from build123d import *

# Parameters (mm, degrees)
SKETCH1_W           = 68
SKETCH1_H           = 54
BOSS_EXTRUDE1_DEPTH = 8
CUT_EXTRUDE1_DEPTH  = 51
SKETCH2_3_W         = 28.5
SKETCH2_3_H         = 2.140954579
SKETCH2_3_W_2       = 28
CUT_EXTRUDE2_DEPTH  = 65.311740763
FILLET1_R           = 3
FILLET2_R           = 3
SKETCH3_W           = 40
SKETCH3_H           = 2.334194627
CUT_EXTRUDE3_DEPTH  = 51
FILLET3_R           = 3
FILLET4_R           = 3
FILLET5_R           = 3
SKETCH1_3_W         = 8
SKETCH1_3_H         = 8
SKETCH1_3_R         = 1.55
BOSS_EXTRUDE2_DEPTH = 3
FILLET6_R           = 3
FILLET7_R           = 1
FILLET8_R           = 1
FILLET9_R           = 1


with BuildPart() as part:
    # Sketch1 → Boss-Extrude1 (new body)
    with BuildSketch(Plane(origin=(0, 0, 0), x_dir=(1, 0, 0), z_dir=(0, 1, 0))):
        Rectangle(SKETCH1_W, SKETCH1_H)
    extrude(amount=BOSS_EXTRUDE1_DEPTH)

    # Sketch2 → Cut-Extrude1 (cut)
    with BuildSketch(Plane(origin=(0, 0, -27), x_dir=(-1, 0, 0), z_dir=(0, 0, -1))):
        Polygon((-30.5, 2.334194627), (0, 2.334194627), (0, 5.859045421), (-28.5, 5.859045421), (-30.5, 5.859045421), align=None)
        Polygon((0, 5.859045421), (0, 2.334194627), (30, 2.334194627), (30, 5.859045421), (28, 5.859045421), align=None)
    extrude(amount=-CUT_EXTRUDE1_DEPTH, mode=Mode.SUBTRACT)

    # Sketch2<3> → Cut-Extrude2 (cut, through all)
    with BuildSketch(Plane(origin=(0, 0, -27), x_dir=(-1, 0, 0), z_dir=(0, 0, -1))):
        with Locations((-14.25, 6.929522711)):
            Rectangle(SKETCH2_3_W, SKETCH2_3_H)
        with Locations((14, 6.929522711)):
            Rectangle(SKETCH2_3_W_2, SKETCH2_3_H)
    extrude(amount=-CUT_EXTRUDE2_DEPTH, mode=Mode.SUBTRACT)

    # Fillet1
    # the kernel refuses this fillet: 3 mm, written as the material it adds along each edge
    with BuildSketch(Plane(origin=(30.5, 5.859045421, -27), x_dir=(0, -1, 0), z_dir=(0, 0, 1))) as fillet1_piece_1:
        with BuildLine():
            CenterArc((2.828427125, -3), FILLET1_R, 90, 70.528779366)
            Line((0, -2), (-0.056568542, -1.98))
            ThreePointArc((-0.056568542, -1.98), (-0.06, -1), (-0.06, 0))
            Line((-0.06, 0), (0, 0.06))
            Line((0, 0.06), (2.828427125, 0.06))
            Line((2.828427125, 0.06), (2.828427125, 0))
        make_face()
    extrude(amount=51)
    with BuildSketch(Plane(origin=(-30, 5.859045421, -27), x_dir=(1, 0, 0), z_dir=(0, 0, 1))) as fillet1_piece_2:
        with BuildLine():
            CenterArc((3, -2.828427125), FILLET1_R, 109.471220634, 70.528779366)
            Line((0, -2.828427125), (-0.06, -2.828427125))
            Line((-0.06, -2.828427125), (-0.06, 0))
            Line((-0.06, 0), (0, 0.06))
            ThreePointArc((0, 0.06), (1, 0.06), (1.98, 0.056568542))
            Line((1.98, 0.056568542), (2, 0))
        make_face()
    extrude(amount=51)

    # Fillet2
    fillet2_edges = [part.edges().sort_by_distance(p)[0] for p in [
        (34, 8, 0),
        (-34, 8, 0),
    ]]
    fillet(fillet2_edges, radius=FILLET2_R)

    # Sketch3 → Cut-Extrude3 (cut)
    with BuildSketch(Plane(origin=(0, 0, -27), x_dir=(-1, 0, 0), z_dir=(0, 0, -1))):
        with Locations((0, 1.167097314)):
            Rectangle(SKETCH3_W, SKETCH3_H)
    extrude(amount=-CUT_EXTRUDE3_DEPTH, mode=Mode.SUBTRACT)

    # Fillet3
    fillet3_edges = [part.edges().sort_by_distance(p)[0] for p in [
        (20, 1.167097313, 24),
        (-20, 1.167097313, 24),
    ]]
    fillet(fillet3_edges, radius=FILLET3_R)

    # Fillet4
    # the kernel refuses this fillet: 3 mm, written as the material it takes off along each edge
    with BuildSketch(Plane(origin=(-17, 2.334194627, 21), x_dir=(0.6464786745536378, 0, -0.762932056835582), z_dir=(-0.762932056835582, 0, -0.6464786745536378))) as fillet4_piece_1_section:
        with BuildLine():
            CenterArc((5.925184303, 3), FILLET4_R, 192.822717627, 77.177282373)
            Line((3, 2.334194627), (3, 0))
            Line((3, 0), (5.925184303, 0))
        make_face()
    fillet4_piece_1 = revolve(axis=Axis((-17, 2.334194627, 21), (0, -1, 0)), revolution_arc=229.72336785, mode=Mode.PRIVATE)
    fillet4_piece_1 = split(fillet4_piece_1, bisect_by=Plane(origin=(-17, 2.334194627, 24), z_dir=(0, 0, -1)), keep=Keep.TOP, mode=Mode.PRIVATE)
    add(fillet4_piece_1, mode=Mode.SUBTRACT)
    with BuildSketch(Plane(origin=(17, 2.334194627, 21), x_dir=(1, 0, 0), z_dir=(0, 0, -1))) as fillet4_piece_2_section:
        with BuildLine():
            CenterArc((5.925184303, 3), FILLET4_R, 192.822717627, 77.177282373)
            Line((3, 2.334194627), (3, 0))
            Line((3, 0), (5.925184303, 0))
        make_face()
    fillet4_piece_2 = revolve(axis=Axis((17, 2.334194627, 21), (0, -1, 0)), revolution_arc=229.72336785, mode=Mode.PRIVATE)
    fillet4_piece_2 = split(fillet4_piece_2, bisect_by=Plane(origin=(17, 2.334194627, 24), z_dir=(0, 0, -1)), keep=Keep.TOP, mode=Mode.PRIVATE)
    add(fillet4_piece_2, mode=Mode.SUBTRACT)
    with BuildSketch(Plane(origin=(-20, 2.334194627, -34.312960757), x_dir=(-1, 0, 0), z_dir=(0, 0, 1))) as fillet4_piece_3:
        with BuildLine():
            CenterArc((2.925184303, 3), FILLET4_R, 192.822717627, 77.177282373)
            Line((0, 2.334194627), (0, 0))
            Line((0, 0), (2.925184303, 0))
        make_face()
    extrude(amount=55.312960757, mode=Mode.SUBTRACT)
    with BuildSketch(Plane(origin=(20, 2.334194627, -34.312960757), x_dir=(1, 0, 0), z_dir=(0, 0, 1))) as fillet4_piece_4:
        with BuildLine():
            CenterArc((2.925184303, -3), FILLET4_R, 90, 77.177282373)
            Line((0, -2.334194627), (0, 0))
            Line((0, 0), (2.925184303, 0))
        make_face()
    extrude(amount=55.312960757, mode=Mode.SUBTRACT)

    # Fillet5
    # the kernel refuses this fillet: 3 mm, written as the material it adds along each edge
    with BuildSketch(Plane(origin=(28.5, 5.859045421, 24), x_dir=(-1, 0, 0), z_dir=(0, 0, 1))) as fillet5_piece_1:
        with BuildLine():
            CenterArc((2.874376622, -3), FILLET5_R, 90, 73.360529794)
            Line((0, -2.140954579), (-0.057487532, -2.123773671))
            ThreePointArc((-0.057487532, -2.123773671), (-0.06, -1.07047729), (-0.06, 0))
            Line((-0.06, 0), (0, 0.06))
            Line((0, 0.06), (2.874376622, 0.06))
            Line((2.874376622, 0.06), (2.874376622, 0))
        make_face()
    extrude(amount=3)
    with BuildSketch(Plane(origin=(-28, 5.859045421, 24), x_dir=(1, 0, 0), z_dir=(0, 0, 1))) as fillet5_piece_2:
        with BuildLine():
            CenterArc((2.874376622, 3), FILLET5_R, 196.639470206, 73.360529794)
            Line((0, 2.140954579), (-0.057487532, 2.123773671))
            ThreePointArc((-0.057487532, 2.123773671), (-0.06, 1.07047729), (-0.06, 0))
            Line((-0.06, 0), (0, -0.06))
            Line((0, -0.06), (2.874376622, -0.06))
            Line((2.874376622, -0.06), (2.874376622, 0))
        make_face()
    extrude(amount=3)

    # Sketch1<3> → Boss-Extrude2 (add)
    # profile 1 of 2: a face of its own
    with BuildSketch(Plane(origin=(0, 0, 0), x_dir=(1, 0, 0), z_dir=(0, 1, 0))):
        with Locations((-38, 0)):
            Rectangle(SKETCH1_3_W, SKETCH1_3_H)
        with Locations(Location((-38, 0, 0), (0, 0, 270))):
            Circle(SKETCH1_3_R, mode=Mode.SUBTRACT)
    # profile 2 of 2: a face of its own
    with BuildSketch(Plane(origin=(0, 0, 0), x_dir=(1, 0, 0), z_dir=(0, 1, 0))):
        with Locations((38, 0)):
            Rectangle(SKETCH1_3_W, SKETCH1_3_H)
        with Locations(Location((38, 0, 0), (0, 0, 270))):
            Circle(SKETCH1_3_R, mode=Mode.SUBTRACT)
    extrude(amount=BOSS_EXTRUDE2_DEPTH)

    # Fillet6
    fillet6_edges = [part.edges().sort_by_distance(p)[0] for p in [
        (-34, 1.5, -4),
        (-34, 1.5, 4),
        (34, 1.5, -4),
        (34, 1.5, 4),
    ]]
    fillet(fillet6_edges, radius=FILLET6_R)

    # Fillet7
    fillet7_edges = [part.edges().sort_by_distance(p)[0] for p in [
        (34, 3, 0),
    ]]
    fillet(fillet7_edges, radius=FILLET7_R)

    # Fillet8
    fillet8_edges = [part.edges().sort_by_distance(p)[0] for p in [
        (-34, 3, 0),
    ]]
    fillet(fillet8_edges, radius=FILLET8_R)

    # Fillet9
    fillet9_edges = [part.edges().sort_by_distance(p)[0] for p in [
        (-42, 1.5, -4),
        (-42, 1.5, 4),
        (42, 1.5, -4),
        (42, 1.5, 4),
    ]]
    fillet(fillet9_edges, radius=FILLET9_R)


solid = part.part
The model under review builds one solid part; all positions refer to its coordinate system, in mm. A direction names the side the tool comes from. Round coordinates to 2 decimals unless told otherwise and drop trailing zeros. Loops run counter-clockwise (first coordinate to the right, second up) from the corner with the lowest first, then second, coordinate; pieces in that order, holes last. Notation, with made-up numbers: (69.5, 48) -> (125.5, 48) arc R21 ccw to (125.5, 54) -> close; hole circle Ø7 at (43, -6.75). An arc over 180 degrees is marked (long way). Answer as CSV lines item,"result".
1) Draft analysis for pull direction X (two halves, no side actions). For faces 1 (the face through (-30, 8, 0)), 2 (the face through (28.5, 7, -2)), 3 (the face through (33.14, 7.1, -0.38)), state which applies: pulls with the +X half, pulls with the -X half, needs draft (parallel to the pull), parting line crosses it, or undercut.
Geometry results:
face 1,"needs draft"
face 2,"undercut"
face 3,"pulls with the +X half"
2) Add section B-B on x = -38. Write out the cut boundary in (y, z).
Geometry results:
outline,"(0, -4) -> (3, -4) -> (3, -1.55) -> (0, -1.55) -> close; (0, 1.55) -> (3, 1.55) -> (3, 4) -> (0, 4) -> close"
3) For P1, Ø6.5, axis at x = 24, z = 3, coming from the +Y side; P2, Ø1.5, axis at y = 5.5, z = 2, coming from the -X side; P3, Ø2, axis at x = 10, y = 6, coming from the -Z side, all flat-tipped, find the tip position at first contact; note any pin that passes through.
Geometry results:
P1,"stops at y = 2.33"
P2,"stops at x = -34"
P3,"stops at z = 24"
4) Add section C-C on z = -14. Write out the cut boundary in (x, y), plus the area to 3 significant figures.
Geometry results:
outline,"(-34, 0) -> (-20, 0) arc R3 ccw to (-22.93, 2.33) -> (-30, 2.33) -> (-30, 3.03) arc R3 cw to (-28, 5.86) -> (-28, 8) -> (-31, 8) arc R3 ccw to (-34, 5) -> close; (20, 0) -> (34, 0) -> (34, 5) arc R3 ccw to (31, 8) -> (28.5, 8) -> (28.5, 5.86) arc R3 cw to (30.5, 3.03) -> (30.5, 2.33) -> (22.93, 2.33) arc R3 ccw to start"
area,"112 mm²"
5) Tool access review of faces 4 (the face through (39, 1, -4)), 5 (the face through (26, 2.334, -2)), 6 (the face through (-39, 1, 4)): name each direction out of +Z, -Z, +X, -X, +Y, -Y from which nothing blocks a thin tool from reaching the whole face with its end or side.
Geometry results:
face 4,"-Z, +X, +Y, -Y"
face 5,"-Z"
face 6,"+Z, -X, +Y, -Y"
6) Add section D-D on x = 27.5. Write out the cut boundary in (y, z).
Geometry results:
outline,"(0, -27) -> (2.33, -27) -> (2.33, 24) -> (6.52, 24) -> (6.52, 27) -> (0, 27) -> close"
7) To check wall thickness, follow line 1 along X through (y, z) = (1.7, 0); line 2 along X through (y, z) = (2.45, 0); line 3 along X through (y, z) = (0.75, -24). State the ranges of each line that lie inside material, in increasing order. Write a range as from..to.
Geometry results:
line 1,"x = -42..-39.55, -36.45..-21.08, 21.08..36.45, 39.55..42"
line 2,"x = -42..-39.55, -36.45..-30, 30.5..36.45, 39.55..42"
line 3,"x = -34..-20.28, 20.28..34"
8) Add section A-A on z = 0. State how many separate pieces and enclosed holes the cut face has, plus the area to 3 significant figures.
Geometry results:
separate pieces,"4"
enclosed holes,"0"
area,"142 mm²"
